The listing builds one solid part. Answer for the finished solid, in the listing's coordinates (mm). A direction names the side the tool comes from. Give positions to 0.01 mm unless a question says otherwise; leave off trailing zeros. Write each loop counter-clockwise with the first axis right and the second up, starting at its lowest first coordinate (ties: lowest second). Pieces come first, ordered by that corner, then holes. Notation, with made-up numbers: (86.5, -35) - (96.5, -35) arc R8 cw to (96.5, -28) - close; hole circle Ø9 at (71.5, -23.5). An arc over 180 degrees is marked (long way). Answer as CSV lines item,"result". Start each with the question number.
(1) Straight lines are drawn through the part: probe 1 along Y at (x, z) = (0, 0.8); probe 2 along X at (y, z) = (-4, 0.5); probe 3 along X at (y, z) = (-14, 2). For each, find the intervals that lie inside material, in ascending order.
(2) Find section A-A (z = 7). State how many separate pieces and enclosed holes the cut face has, then the cut area to 3 significant figures.
(3) Each of these flat-tipped pins is pushed along its axis until it touches: pin 1 Ø6 at (x, y) = (18.5, -5.5) entering from +Z; pin 2 Ø0.6 at (y, z) = (-11.5, 1) entering from +X; pin 3 Ø2 at (x, z) = (15.5, 3) entering from +Y; pin 4 Ø23 at (x, y) = (0, 0) entering from +Z. Where does it stop, or does it pass through?
(4) For faces 1 (the face through (11, 0, 4)), 2 (the face through (7.1, -18.3, 10.75)), 3 (the face through (0, 13, 1)), determine the directions among +Z, -Z, +X, -X, +Y, -Y from which every point of the face is accessible in a straight line to the end or side of a thin tool.
(5) Find section B-B (y = 17). Write down the section's boundary in (x, z).
(6) Find section D-D (y = -1). Write down the section's boundary in (x, z), then the cut area to 3 significant figures.
(7) For a pull along Y with two mould halves and no side action, classify faces 4 (the face through (2.8, -12.65, 2.77)), 5 (the face through (16, 14, 10.75)) as pulls with the +Y half, pulls with the -Y half, needs draft (parallel to the pull), parting line crosses it, or undercut.
from build123d import *

# Parameters (mm, degrees)
SKETCH1_R           = 25
SKETCH1_R_2         = 8.75
BOSS_EXTRUDE1_DEPTH = 4
SKETCH2_R           = 5
SKETCH2_R_2         = 2
BOSS_EXTRUDE2_DEPTH = 6.75
CUT_EXTRUDE1_START  = -6.75
SKETCH5_R           = 2
CUT_EXTRUDE1_DEPTH  = 6.75
CUT_EXTRUDE2_DEPTH  = 2.5


with BuildPart() as part:
    # Sketch1 → Boss-Extrude1 (new body)
    with BuildSketch(Plane.XY):
        Circle(SKETCH1_R)
        Circle(SKETCH1_R_2, mode=Mode.SUBTRACT)
        with BuildLine():
            Line((-1.5, 11), (-1.5, 11.5))
            ThreePointArc((-1.5, 11.5), (0, 13), (1.5, 11.5))
            Line((1.5, 11.5), (1.5, 11))
            ThreePointArc((1.5, 11), (0, 9.5), (-1.5, 11))
        make_face(mode=Mode.SUBTRACT)
        with BuildLine():
            Line((-1.5, -11), (-1.5, -11.5))
            ThreePointArc((-1.5, -11.5), (0, -13), (1.5, -11.5))
            Line((1.5, -11.5), (1.5, -11))
            ThreePointArc((1.5, -11), (0, -9.5), (-1.5, -11))
        make_face(mode=Mode.SUBTRACT)
    extrude(amount=BOSS_EXTRUDE1_DEPTH)

    # Sketch2 → Boss-Extrude2 (add)
    # profile 1 of 6: a face of its own
    with BuildSketch(Plane.XY.offset(4)):
        with Locations((-4.917561857, 18.352590699)):
            Circle(SKETCH2_R)
        with Locations((-4.917561857, 18.352590699)):
            Circle(SKETCH2_R_2, mode=Mode.SUBTRACT)
    # profile 2 of 6: a face of its own
    with BuildSketch(Plane.XY.offset(4)):
        with Locations((-18.352590699, 4.917561857)):
            Circle(SKETCH2_R)
        with Locations((-18.352590699, 4.917561857)):
            Circle(SKETCH2_R_2, mode=Mode.SUBTRACT)
    # profile 3 of 6: a face of its own
    with BuildSketch(Plane.XY.offset(4)):
        with Locations((-13.435028843, -13.435028843)):
            Circle(SKETCH2_R)
        with Locations((-13.435028843, -13.435028843)):
            Circle(SKETCH2_R_2, mode=Mode.SUBTRACT)
    # profile 4 of 6: a face of its own
    with BuildSketch(Plane.XY.offset(4)):
        with Locations((4.917561857, -18.352590699)):
            Circle(SKETCH2_R)
        with Locations((4.917561857, -18.352590699)):
            Circle(SKETCH2_R_2, mode=Mode.SUBTRACT)
    # profile 5 of 6: a face of its own
    with BuildSketch(Plane.XY.offset(4)):
        with Locations((18.352590699, -4.917561857)):
            Circle(SKETCH2_R)
        with Locations((18.352590699, -4.917561857)):
            Circle(SKETCH2_R_2, mode=Mode.SUBTRACT)
    # profile 6 of 6: a face of its own
    with BuildSketch(Plane.XY.offset(4)):
        with Locations((13.435028843, 13.435028843)):
            Circle(SKETCH2_R)
        with Locations((13.435028843, 13.435028843)):
            Circle(SKETCH2_R_2, mode=Mode.SUBTRACT)
    extrude(amount=BOSS_EXTRUDE2_DEPTH)

    # Sketch5 → Cut-Extrude1 (cut)
    with BuildSketch(Plane.XY.offset(4).offset(CUT_EXTRUDE1_START)):
        with Locations((-18.352590699, 4.917561857)):
            Circle(SKETCH5_R)
        with Locations((-13.435028843, -13.435028843)):
            Circle(SKETCH5_R)
        with Locations((4.917561857, -18.352590699)):
            Circle(SKETCH5_R)
        with Locations((18.352590699, -4.917561857)):
            Circle(SKETCH5_R)
        with Locations((13.435028843, 13.435028843)):
            Circle(SKETCH5_R)
        with Locations((-4.917561857, 18.352590699)):
            Circle(SKETCH5_R)
    extrude(amount=CUT_EXTRUDE1_DEPTH, mode=Mode.SUBTRACT)

    # Sketch6 → Cut-Extrude2 (cut)
    with BuildSketch(Plane.XY.offset(4)):
        Polygon((1.876388375, -7.75), (-1.876388375, -7.75), (-3.75277675, -11), (-1.876388375, -14.25), (1.876388375, -14.25), (3.75277675, -11), align=None)
        Polygon((1.876388375, 14.25), (3.75277675, 11), (1.876388375, 7.75), (-1.876388375, 7.75), (-3.75277675, 11), (-1.876388375, 14.25), align=None)
    extrude(amount=-CUT_EXTRUDE2_DEPTH, mode=Mode.SUBTRACT)


solid = part.part
Result set:
1,probe 1,"-25 to -13, -9.5 to -8.75, 8.75 to 9.5, 13 to 25"
1,probe 2,"-24.68 to -7.78, 7.78 to 16.58, 20.13 to 24.68"
1,probe 3,"-20.71 to -15.35, -11.52 to -2.02, 2.02 to 20.71"
2,separate pieces,"6"
2,enclosed holes,"6"
2,area,"396 mm^2"
3,pin 1,"z = 10.75"
3,pin 2,"x = 22.35"
3,pin 3,"y = 20.37"
3,pin 4,"z = 4"
4,face 1,"+Z"
4,face 2,"+Z, +X, -X, +Y, -Y"
4,face 3,"+Z, -Z"
5,outline,"(-18.33, 0) - (-6.39, 0) - (-6.39, 10.75) - (-9.73, 10.75) - (-9.73, 4) - (-18.33, 4) - close; (-3.44, 0) - (18.33, 0) - (18.33, 4) - (16.94, 4) - (16.94, 10.75) - (9.93, 10.75) - (9.93, 4) - (-0.1, 4) - (-0.1, 10.75) - (-3.44, 10.75) - close"
6,outline,"(-24.98, 0) - (-8.69, 0) - (-8.69, 4) - (-24.98, 4) - close; (8.69, 0) - (24.98, 0) - (24.98, 4) - (21.46, 4) - (21.46, 10.75) - (15.25, 10.75) - (15.25, 4) - (8.69, 4) - close"
6,area,"172 mm^2"
7,face 4,"undercut"
7,face 5,"needs draft"
